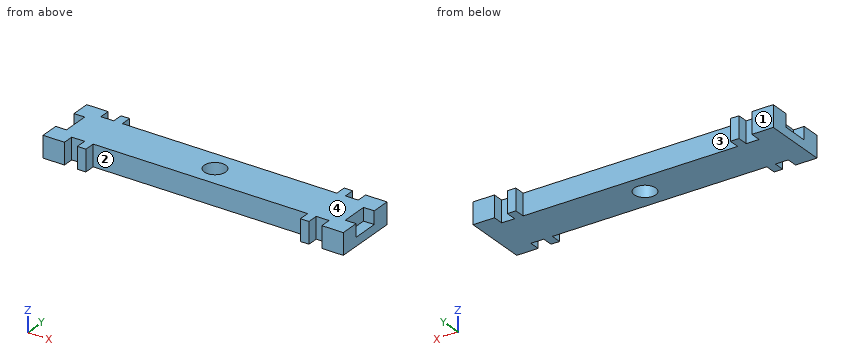
```python
from build123d import *

# Parameters (mm, degrees)
F0_R     = 5
F1_DEPTH = 10
F2_W     = 10
F2_H     = 12.5
F3_DEPTH = 6


with BuildPart() as f1:
    # F0 (on Top) → F1 (new body)
    with BuildSketch(Plane.XY):
        Polygon((-50, -10), (50, -10), (50, -15), (54, -15), (54, -10), (60, -10), (60, -15), (70, -15), (70, 0), (70, 15), (60, 15), (60, 10), (54, 10), (54, 15), (50, 15), (50, 10), (-50, 10), (-50, 15), (-54, 15), (-54, 10), (-60, 10), (-60, 15), (-70, 15), (-70, 0), (-70, -15), (-60, -15), (-60, -10), (-54, -10), (-54, -15), (-50, -15), align=None)
        Circle(F0_R, mode=Mode.SUBTRACT)
    extrude(amount=F1_DEPTH)

    # F2 (on face) → F3 (cut)
    with BuildSketch(Plane.XY.offset(10)):
        with Locations((70, 0)):
            Rectangle(F2_W, F2_H)
        with Locations((-70, 0)):
            Rectangle(F2_W, F2_H)
    extrude(amount=-F3_DEPTH, mode=Mode.SUBTRACT)


solid = f1.part
```
For this review, take the finished solid that the model builds, in its own axes (mm). Face numbers are marked on the shaded views. A direction names the side the tool comes from. Round coordinates to 2 decimals unless told otherwise and drop trailing zeros. Write each loop counter-clockwise with the first axis right and the second up, starting at its lowest first coordinate (ties: lowest second). Pieces come first, ordered by that corner, then holes. Notation, with made-up numbers: (-0.5, 77) -> (39.5, 77) arc R26 ccw to (39.5, 116) -> close; hole circle Ø6 at (-12.5, -23). An arc over 180 degrees is marked (long way). One line per question, with ' | ' between items. Start each with the question number.
1) Add section A-A (y = 11.5). Write out the cut boundary in (x, z), and give its area (3 significant figures).
2) Machinability: for the marked faces 3 and 4, which of the approach directions +Z, -Z, +X, -X, +Y, -Y give a long, thin tool a straight path to every point of the face, cutting with its end or side? Answer none if there is none.
3) Wall thickness on line 1 along Y through (x, z) = (0, 8.25); line 2 along Y through (x, z) = (59.5, 7.25); line 3 along X through (y, z) = (2.5, 4.5): over which ranges is each line inside the solid? List them lowest first.
4) Add section D-D (x = 3). Write out the cut boundary in (y, z).
5) Mouldability with a two-part tool opening along X and no side actions: class the marked faces 1 and 2 as +X half, -X half, draft (parallel to the pull), parting line (faces both ways), or undercut.
6) For pin 1 Ø1.8 at (x, z) = (-56.5, 7.5) entering from +Y; pin 2 Ø4 at (x, z) = (-28, 5.5) entering from -Y; pin 3 Ø4 at (x, y) = (67.5, 3) entering from +Z, all flat-tipped, find the tip position at first contact; note any pin that passes through.
7) Add section C-C (y = -3). Write out the cut boundary in (x, z), and give its area (3 significant figures).
Reported:
1) outline: (-70, 0) -> (-60, 0) -> (-60, 10) -> (-70, 10) -> close; (-54, 0) -> (-50, 0) -> (-50, 10) -> (-54, 10) -> close; (50, 0) -> (54, 0) -> (54, 10) -> (50, 10) -> close; (60, 0) -> (70, 0) -> (70, 10) -> (60, 10) -> close | area: 280 mm²
2) face 3: +Z, -Z, +Y | face 4: +Z, +X, -X, +Y, -Y
3) line 1: y = -10 to -5, 5 to 10 | line 2: y = -10 to 10 | line 3: x = -65 to -4.33, 4.33 to 65
4) outline: (-10, 0) -> (-4, 0) -> (-4, 10) -> (-10, 10) -> close; (4, 0) -> (10, 0) -> (10, 10) -> (4, 10) -> close
5) face 1: draft | face 2: undercut
6) pin 1: stops at y = 10 | pin 2: stops at y = -10 | pin 3: stops at z = 4
7) outline: (-70, 0) -> (-4, 0) -> (-4, 10) -> (-65, 10) -> (-65, 4) -> (-70, 4) -> close; (4, 0) -> (70, 0) -> (70, 4) -> (65, 4) -> (65, 10) -> (4, 10) -> close | area: 1,260 mm²
